The listing builds one solid part. Answer for the finished solid, in the listing's coordinates (mm). Coordinates: 2 decimals unless noted, no trailing zeros. Write each loop counter-clockwise with the first axis right and the second up, starting at its lowest first coordinate (ties: lowest second). Pieces come first, ordered by that corner, then holes.
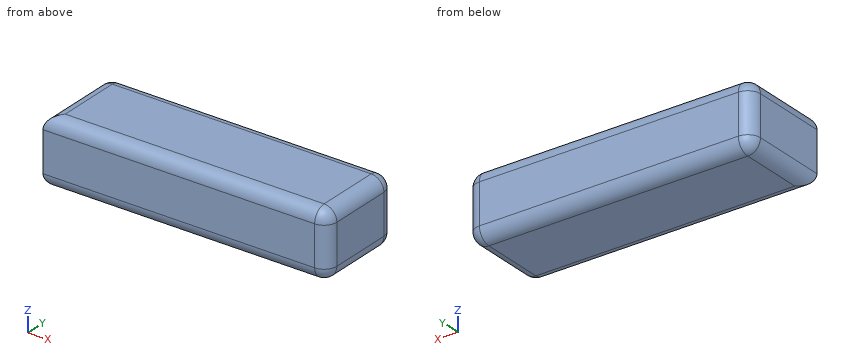
from build123d import *

# Parameters (mm, degrees)
SKETCH1_W           = 156
SKETCH1_H           = 49
BOSS_EXTRUDE1_DEPTH = 36
FILLET1_R           = 7


with BuildPart() as part:
    # Sketch1 → Boss-Extrude1 (new body)
    with BuildSketch(Plane.XY):
        with Locations((78, 24.5)):
            Rectangle(SKETCH1_W, SKETCH1_H)
    extrude(amount=BOSS_EXTRUDE1_DEPTH)

    # Fillet1
    fillet1_edges = [part.edges().sort_by_distance(p)[0] for p in [
        (156, 24.5, 36),
        (78, 49, 36),
        (0, 24.5, 36),
        (78, 49, 0),
        (156, 24.5, 0),
        (78, 0, 0),
        (0, 24.5, 0),
        (78, 0, 36),
        (0, 49, 18),
        (156, 49, 18),
        (156, 0, 18),
    ]]
    fillet(fillet1_edges, radius=FILLET1_R)


solid = part.part
1. Find the intervals of material crossed by L1, parallel to Z at x = 18.5, y = 2.5; L2, parallel to Z at x = 103.5, y = 45; L3, parallel to X at y = 21.5, z = 3.5, in increasing order.
Results found:
L1: z = 1.64 to 34.36
L2: z = 0.68 to 35.32
L3: x = 0.94 to 155.06
2. Section C-C on z = 4 is taken. Give the vertices of the cut face in (x, y).
Results found:
outline: (0.68, 0.68) - (149, 0.68) arc R6.32 ccw to (155.32, 7) - (155.32, 42) arc R6.32 ccw to (149, 48.32) - (7, 48.32) arc R6.32 ccw to (0.68, 42) - close
3. Section A-A on x = 111 is taken. Give the vertices of the cut face in (y, z), then the cut area to 3 significant figures.
Results found:
outline: (0, 7) arc R7 ccw to (7, 0) - (42, 0) arc R7 ccw to (49, 7) - (49, 29) arc R7 ccw to (42, 36) - (7, 36) arc R7 ccw to (0, 29) - close
area: 1,720 mm2
4. Section B-B on z = 31.5 is taken. Give the vertices of the cut face in (x, y), then the cut area to 3 significant figures.
Results found:
outline: (0.46, 0.46) - (149, 0.46) arc R6.54 ccw to (155.54, 7) - (155.54, 42) arc R6.54 ccw to (149, 48.54) - (7, 48.54) arc R6.54 ccw to (0.46, 42) - close
area: 7,430 mm2
